```python
from build123d import *

# Parameters (mm, degrees)
SKETCH_1_W           = 150
SKETCH_1_H           = 150
EXTRUDE_1_DEPTH      = 10
SKETCH_2_R           = 13
CUT_EXTRUDE_1_DEPTH  = 8
SKETCH_3_R           = 7.5
CUT_EXTRUDE_3_DEPTH  = 213.367605816
SKETCH_4_R           = 22
CUT_EXTRUDE_4_DEPTH  = 2
SKETCH_5_R           = 2.5
CUT_EXTRUDE_5_DEPTH  = 213.367605816
SKETCH_6_W           = 163.457358394
SKETCH_6_H           = 157.320035801
SKETCH_6_W_2         = 146.6
SKETCH_6_H_2         = 146.6
CUT_EXTRUDE_6_DEPTH  = 7
SKETCH_7_R           = 1.65
CUT_EXTRUDE_7_DEPTH  = 15
CUT_EXTRUDE_START    = -15
SKETCH_8_R           = 1.65
CUT_EXTRUDE_8_DEPTH  = 15
SKETCH_9_R           = 1.65
CUT_EXTRUDE_9_DEPTH  = 15
SKETCH_10_R          = 1.65
CUT_EXTRUDE_10_DEPTH = 15
SKETCH_12_R          = 1.25
CUT_EXTRUDE_11_DEPTH = 213.367605816
SKETCH_14_R          = 5
CUT_EXTRUDE_12_DEPTH = 5
SKETCH_15_W          = 100
SKETCH_15_H          = 50
CUT_EXTRUDE_13_DEPTH = 2
SKETCH_16_R          = 7.1
CUT_EXTRUDE_14_DEPTH = 2
SKETCH_17_R          = 3
CUT_EXTRUDE_15_DEPTH = 213.367605816
SKETCH_18_W          = 20
SKETCH_18_H          = 10
CUT_EXTRUDE_16_DEPTH = 2
CUT_EXTRUDE_17_DEPTH = 4
SKETCH_20_R          = 1.35
CUT_EXTRUDE_18_DEPTH = 4


with BuildPart() as part:
    # Эскиз1 → Бобышка-Вытянуть1 (new body)
    with BuildSketch(Plane.XY):
        with Locations((75, 75)):
            Rectangle(SKETCH_1_W, SKETCH_1_H)
    extrude(amount=EXTRUDE_1_DEPTH)

    # Эскиз2 → Вырез-Вытянуть1 (cut)
    with BuildSketch(Plane.XY.offset(10)):
        with Locations((75, 37)):
            Circle(SKETCH_2_R)
    extrude(amount=-CUT_EXTRUDE_1_DEPTH, mode=Mode.SUBTRACT)

    # Эскиз3 → Вырез-Вытянуть3 (cut, through all)
    with BuildSketch(Plane.XY.offset(10)):
        with Locations((75, 37)):
            Circle(SKETCH_3_R)
    extrude(amount=-CUT_EXTRUDE_3_DEPTH, mode=Mode.SUBTRACT)

    # Эскиз4 → Вырез-Вытянуть4 (cut)
    with BuildSketch(Plane.XY.offset(10)):
        with Locations((75, 37)):
            Circle(SKETCH_4_R)
    extrude(amount=-CUT_EXTRUDE_4_DEPTH, mode=Mode.SUBTRACT)

    # Эскиз5 → Вырез-Вытянуть5 (cut, through all)
    with BuildSketch(Plane.XY.offset(10)):
        with Locations((51.43, 13.43)):
            Circle(SKETCH_5_R)
        with Locations((98.57, 13.43)):
            Circle(SKETCH_5_R)
        with Locations((98.57, 60.57)):
            Circle(SKETCH_5_R)
        with Locations((51.43, 60.57)):
            Circle(SKETCH_5_R)
    extrude(amount=-CUT_EXTRUDE_5_DEPTH, mode=Mode.SUBTRACT)

    # Эскиз6 → Вырез-Вытянуть6 (cut)
    with BuildSketch(Plane(origin=(0, 0, 0), x_dir=(-1, 0, 0), z_dir=(0, 0, -1))):
        with Locations((-77.352640327, 75.40915484)):
            Rectangle(SKETCH_6_W, SKETCH_6_H)
        with Locations((-75, 75)):
            Rectangle(SKETCH_6_W_2, SKETCH_6_H_2, mode=Mode.SUBTRACT)
    extrude(amount=-CUT_EXTRUDE_6_DEPTH, mode=Mode.SUBTRACT)

    # Эскиз7 → Вырез-Вытянуть7 (cut)
    with BuildSketch(Plane.XZ.offset(-1.7)):
        with Locations(Location((20, 3.5, 0), (0, 0, 270))):
            Circle(SKETCH_7_R)
        with Locations(Location((75, 3.5, 0), (0, 0, 270))):
            Circle(SKETCH_7_R)
        with Locations(Location((130, 3.5, 0), (0, 0, 270))):
            Circle(SKETCH_7_R)
    extrude(amount=-CUT_EXTRUDE_7_DEPTH, mode=Mode.SUBTRACT)

    # Эскиз8 → Вырез-Вытянуть8 (cut)
    with BuildSketch(Plane(origin=(0, 148.3, 0), x_dir=(1, 0, 0), z_dir=(0, 1, 0)).offset(CUT_EXTRUDE_START)):
        with Locations(Location((20, -3.5, 0), (0, 0, 90))):
            Circle(SKETCH_8_R)
        with Locations(Location((75, -3.5, 0), (0, 0, 90))):
            Circle(SKETCH_8_R)
        with Locations(Location((130, -3.5, 0), (0, 0, 90))):
            Circle(SKETCH_8_R)
    extrude(amount=CUT_EXTRUDE_8_DEPTH, mode=Mode.SUBTRACT)

    # Эскиз9 → Вырез-Вытянуть9 (cut)
    with BuildSketch(Plane(origin=(148.3, 0, 0), x_dir=(0, 0, -1), z_dir=(1, 0, 0))):
        with Locations(Location((-3.5, 21.7, 0), (0, 0, 90))):
            Circle(SKETCH_9_R)
        with Locations(Location((-3.5, 128.3, 0), (0, 0, 90))):
            Circle(SKETCH_9_R)
        with Locations(Location((-3.5, 75, 0), (0, 0, 90))):
            Circle(SKETCH_9_R)
    extrude(amount=-CUT_EXTRUDE_9_DEPTH, mode=Mode.SUBTRACT)

    # Эскиз10 → Вырез-Вытянуть10 (cut)
    with BuildSketch(Plane.ZY.offset(-1.7).offset(CUT_EXTRUDE_START)):
        with Locations(Location((3.5, 128.3, 0), (0, 0, 90))):
            Circle(SKETCH_10_R)
        with Locations(Location((3.5, 75, 0), (0, 0, 90))):
            Circle(SKETCH_10_R)
        with Locations(Location((3.5, 21.7, 0), (0, 0, 90))):
            Circle(SKETCH_10_R)
    extrude(amount=CUT_EXTRUDE_10_DEPTH, mode=Mode.SUBTRACT)

    # Эскиз12 → Вырез-Вытянуть11 (cut, through all)
    with BuildSketch(Plane.XY.offset(10)):
        with Locations((75, 20)):
            Circle(SKETCH_12_R)
        with Locations((60.277568136, 45.5)):
            Circle(SKETCH_12_R)
        with Locations((89.722431864, 45.5)):
            Circle(SKETCH_12_R)
        with Locations((58, 37)):
            Circle(SKETCH_12_R)
        with Locations((83.5, 22.277568136)):
            Circle(SKETCH_12_R)
        with Locations((83.5, 51.722431864)):
            Circle(SKETCH_12_R)
    extrude(amount=-CUT_EXTRUDE_11_DEPTH, mode=Mode.SUBTRACT)

    # Эскиз14 → Вырез-Вытянуть12 (cut)
    with BuildSketch(Plane.XY.offset(10)):
        with Locations((51.43, 13.43)):
            Circle(SKETCH_14_R)
        with Locations((98.57, 13.43)):
            Circle(SKETCH_14_R)
        with Locations((98.57, 60.57)):
            Circle(SKETCH_14_R)
        with Locations((51.43, 60.57)):
            Circle(SKETCH_14_R)
    extrude(amount=-CUT_EXTRUDE_12_DEPTH, mode=Mode.SUBTRACT)

    # Эскиз15 → Вырез-Вытянуть13 (cut)
    with BuildSketch(Plane.XY.offset(10)):
        with Locations((75, 115)):
            Rectangle(SKETCH_15_W, SKETCH_15_H)
    extrude(amount=-CUT_EXTRUDE_13_DEPTH, mode=Mode.SUBTRACT)

    # Эскиз16 → Вырез-Вытянуть14 (cut)
    with BuildSketch(Plane.XY.offset(10)):
        with Locations((29.5, 94.5)):
            Circle(SKETCH_16_R)
        with Locations((120.5, 94.5)):
            Circle(SKETCH_16_R)
    extrude(amount=-CUT_EXTRUDE_14_DEPTH, mode=Mode.SUBTRACT)

    # Эскиз17 → Вырез-Вытянуть15 (cut, through all)
    with BuildSketch(Plane.XY.offset(10)):
        with Locations((75, 115)):
            Circle(SKETCH_17_R)
    extrude(amount=-CUT_EXTRUDE_15_DEPTH, mode=Mode.SUBTRACT)

    # Эскиз18 → Вырез-Вытянуть16 (cut)
    with BuildSketch(Plane.XY.offset(10)):
        with Locations((35, 145)):
            Rectangle(SKETCH_18_W, SKETCH_18_H)
        with Locations((115, 145)):
            Rectangle(SKETCH_18_W, SKETCH_18_H)
    extrude(amount=-CUT_EXTRUDE_16_DEPTH, mode=Mode.SUBTRACT)

    # Эскиз19 → Вырез-Вытянуть17 (cut)
    with BuildSketch(Plane(origin=(0, 0, 0), x_dir=(-1, 0, 0), z_dir=(0, 0, -1))):
        Polygon((-69.226497308, 115), (-72.113248654, 120), (-77.886751346, 120), (-80.773502692, 115), (-77.886751346, 110), (-72.113248654, 110), align=None)
    extrude(amount=-CUT_EXTRUDE_17_DEPTH, mode=Mode.SUBTRACT)

    # Эскиз20 → Вырез-Вытянуть18 (cut)
    with BuildSketch(Plane(origin=(0, 0, 0), x_dir=(-1, 0, 0), z_dir=(0, 0, -1))):
        with Locations((-70.397013545, 115)):
            Circle(SKETCH_20_R)
        with Locations((-72.698506772, 111.013696796)):
            Circle(SKETCH_20_R)
        with Locations((-77.301493228, 111.013696796)):
            Circle(SKETCH_20_R)
        with Locations((-79.602986455, 115)):
            Circle(SKETCH_20_R)
        with Locations((-77.301493228, 118.986303204)):
            Circle(SKETCH_20_R)
        with Locations((-72.698506772, 118.986303204)):
            Circle(SKETCH_20_R)
    extrude(amount=-CUT_EXTRUDE_18_DEPTH, mode=Mode.SUBTRACT)


solid = part.part
```
The model under review builds one solid part; all positions refer to its coordinate system, in mm. A direction names the side the tool comes from. Round coordinates to 2 decimals unless told otherwise and drop trailing zeros. Order: outer loops, then holes, each group sorted by start corner. A loop starts at its lowest first (then second) coordinate and runs counter-clockwise, first axis right, second up. Notation, with made-up numbers: (11, 26.25) - (44, 26.25) arc R35 ccw to (44, 59.25) - close; hole circle Ø6 at (-21, 75.25). An arc over 180 degrees is marked (long way). Answer in a Markdown table with one row per item.
(1) Machinability: for faces 1 (the face through (140.9, 20.05, 3.57)), 2 (the face through (75, 16.7, 4)), 3 (the face through (53.737, 56.134, 7.535)), 4 (the face through (76, 1.7, 5)), which of the approach directions +Z, -Z, +X, -X, +Y, -Y give a long, thin tool a straight path to every point of the face, cutting with its end or side? Answer none if there is none.
Result set:
| item | result |
|---|---|
| face 1 | +X |
| face 2 | -Y |
| face 3 | +Z |
| face 4 | -Z, +X, -X, -Y |
(2) Take a section at A-A on x = 141. Write out the cut boundary in (y, z), plus the area to 3 significant figures.
Result set:
| item | result |
|---|---|
| outline | (0, 7) - (1.7, 7) - (1.7, 0) - (148.3, 0) - (148.3, 7) - (150, 7) - (150, 10) - (0, 10) - close; hole circle Ø3.3 at (21.7, 3.5); hole circle Ø3.3 at (75, 3.5); hole circle Ø3.3 at (128.3, 3.5) |
| area | 1,450 mm2 |
(3) Clearance check with flat-ended pins moving along their axes: P1, Ø3, axis at x = 75, z = 3.5, coming from the -Y side; P2, Ø1, axis at x = 129.5, z = 4, coming from the +Y side; P3, Ø1, axis at x = 45.5, z = 2.5, coming from the +Y side; P4, Ø4, axis at x = 51.43, y = 60.57, coming from the +Z side. State where each tip first meets the part, or that it passes through.
Result set:
| item | result |
|---|---|
| P1 | stops at y = 16.7 |
| P2 | stops at y = 133.3 |
| P3 | stops at y = 148.3 |
| P4 | passes through |
(4) For line 1 (X direction, y = 137.75, z = 3.5); line 2 (Y direction, x = 75, z = 3.9); line 3 (X direction, y = 107.5, z = 9), list the stretches that pass through material, from the lowest coordinate up. Write a range as from..to.
Result set:
| item | result |
|---|---|
| line 1 | x = 1.7..18.35, 21.65..73.35, 76.65..128.35, 131.65..148.3 |
| line 2 | y = 16.7..18.75, 21.25..24, 50..110, 120..133.3 |
| line 3 | x = 0..25, 125..150 |
(5) Mouldability with a two-part tool opening along Z and no side actions: class faces 5 (the face through (48.932, 60.68, 2.535)), 6 (the face through (130, 133.3, 4)), 7 (the face through (81, 31, 2)) as released by +Z, released by -Z, zero draft, split by the parting line, or undercut.
Result set:
| item | result |
|---|---|
| face 5 | zero draft |
| face 6 | undercut |
| face 7 | released by +Z |
(6) Take a section at C-C on x = 120.5. Write out the cut boundary in (y, z), plus the area to 3 significant figures.
Result set:
| item | result |
|---|---|
| outline | (0, 7) - (1.7, 7) - (1.7, 0) - (148.3, 0) - (148.3, 7) - (150, 7) - (150, 8) - (87.4, 8) - (87.4, 10) - (0, 10) - close |
| area | 1,350 mm2 |
(7) Take a section at D-D on y = 102. Write out the cut boundary in (x, z), plus the area to 3 significant figures.
Result set:
| item | result |
|---|---|
| outline | (0, 7) - (1.7, 7) - (1.7, 0) - (148.3, 0) - (148.3, 7) - (150, 7) - (150, 10) - (125, 10) - (125, 8) - (25, 8) - (25, 10) - (0, 10) - close |
| area | 1,280 mm2 |
(8) Take a section at B-B on y = 137. Write out the cut boundary in (x, z), plus the area to 3 significant figures.
Result set:
| item | result |
|---|---|
| outline | (0, 7) - (1.7, 7) - (1.7, 0) - (148.3, 0) - (148.3, 7) - (150, 7) - (150, 10) - (125, 10) - (125, 8) - (25, 8) - (25, 10) - (0, 10) - close; hole circle Ø3.3 at (20, 3.5); hole circle Ø3.3 at (75, 3.5); hole circle Ø3.3 at (130, 3.5) |
| area | 1,250 mm2 |
